```python
from build123d import *

# Parameters (mm, degrees)
PAD_DEPTH    = 0.25
PAD001_DEPTH = 0.5


with BuildPart() as part:
    # Sketch → Pad (new body, symmetric)
    with BuildSketch(Plane.XY):
        with BuildLine():
            Line((-0.375, 0), (0, 0))
            Line((0, 0), (0.375, 0))
            ThreePointArc((0.375, 0), (9.051962, -20.948038), (30, -29.625))
            Line((30, -29.625), (30, -30.375))
            ThreePointArc((-0.375, 0), (8.521632, -21.478368), (30, -30.375))
        make_face()
    extrude(amount=PAD_DEPTH, both=True)

    # Sketch002 → Pad001 (join)
    with BuildSketch(Plane.XZ):
        with BuildLine():
            ThreePointArc((-1.25, 0.75), (-1.426777, 0.676777), (-1.5, 0.5))
            Line((-1.5, -0.5), (-1.5, 0.5))
            ThreePointArc((-1.5, -0.5), (-1.426777, -0.676777), (-1.25, -0.75))
            Line((1.25, -0.75), (-1.25, -0.75))
            ThreePointArc((1.25, -0.75), (1.426777, -0.676777), (1.5, -0.5))
            Line((1.5, 0.5), (1.5, -0.5))
            ThreePointArc((1.5, 0.5), (1.426777, 0.676777), (1.25, 0.75))
            Line((-1.25, 0.75), (1.25, 0.75))
        make_face()
    extrude(amount=PAD001_DEPTH)

    # Sketch003 (on DatumPlane) → Revolution (revolve)
    with BuildSketch(Plane(origin=(30, -30, 0), x_dir=(1, 0, 0), z_dir=(0, 0, 1))):
        with BuildLine():
            Line((0, 0), (-0.1825, 0))
            Line((-0.1825, 0), (-0.1825, 0.75))
            Line((-0.1825, 0.75), (0.3175, 0.75))
            Line((0.3175, 0.75), (0.3175, 0.549926))
            ThreePointArc((0.3175, 0.549926), (0.085074, 0.3175), (0, 0))
        make_face()
    revolve(axis=Axis((30, -30, 0), (-1, 0, 0)))


solid = part.part
```
Could you check a few things on this model? Use its own coordinates, in mm. A direction names the side the tool comes from. Round coordinates to 2 decimals unless told otherwise and drop trailing zeros. Write each loop counter-clockwise with the first axis right and the second up, starting at its lowest first coordinate (ties: lowest second). Pieces come first, ordered by that corner, then holes. Notation, with made-up numbers: M 50,23 L 101,23 A17 ccw 101,33 Z; hole C 80.5,-39 d5. An arc over 180 degrees is marked long. Write each question's results on one line, items separated by ' | '. Start each with the question number.
1. Imagine slicing it at B-B on x = 4. List the corners of the cut face in (y, z) for me.
2. On a 3-axis mill with a long thin cutter (end or side, diameter ignored), from which of +Z, -Z, +X, -X, +Y, -Y can I reach the whole of each face in a straight line? I mean faces 1 (the face through (11, -23, 0.25)), 2 (the face through (11, -23, -0.25)), 3 (the face through (0, 0, 0)). Say none if no direction works.
3. I need wall thicknesses on L1, parallel to X at y = -24, z = 0.1; L2, parallel to Y at x = 22.5, z = -0.2; L3, parallel to X at y = -16, z = 0. Which ranges of each line are inside material? Lowest first, please. Write a range as from..to.
4. I'm going to push flat-ended pins straight in: pin 1 Ø5 at (x, y) = (6, -13.5) entering from +Z; pin 2 Ø10 at (x, y) = (15, -15) entering from +Z. Where does each tip first touch, or does it pass through?
Result sheet:
1) outline: M -15.7,-0.25 L -14.2,-0.25 L -14.2,0.25 L -15.7,0.25 Z
2) face 1: +Z, -X, -Y | face 2: -Z, -X, -Y | face 3: +Z, -Z, +X, -X, +Y
3) L1: x = 11.38..12.63 | L2: y = -29.43..-28.66 | L3: x = 4.18..5.07
4) pin 1: stops at z = 0.25 | pin 2: passes through
